Can you work these out from the model? Positions are in its coordinate system, mm. Face numbers are marked on the shaded views. A direction names the side the tool comes from. Give positions to 0.01 mm unless a question says otherwise; leave off trailing zeros. Loops run counter-clockwise (first coordinate to the right, second up) from the corner with the lowest first, then second, coordinate; pieces in that order, holes last. Notation, with made-up numbers: (28, 85) - (59, 85) arc R30 ccw to (59, 110) - close; hole circle Ø10 at (-0.5, 76). An arc over 180 degrees is marked (long way). Answer in a Markdown table with one row per item.
from build123d import *

# Parameters (mm, degrees)
SKETCH1_R                 = 1.75
BASE_DEPTH                = 2
SKETCH2_W                 = 7
SKETCH2_H                 = 16
SIDE_BATTERY_GUIDES_DEPTH = 14
CUT_EXTRUDE1_DEPTH        = 50.658836072
SKETCH5_W                 = 15
SKETCH5_H                 = 2.5
BOSS_EXTRUDE3_DEPTH       = 6
CUT_EXTRUDE2_DEPTH        = 44.33589736
FILLET2_R                 = 2
SKETCH7_R                 = 1.6
CUT_EXTRUDE3_DEPTH        = 44.33589736
SKETCH8_W                 = 26
SKETCH8_H                 = 18
SKETCH8_R                 = 1.75
PINOUT_BD_HOLDER_DEPTH    = 2
WEIGH_REDUCER_DEPTH       = 53.318734694
FILLET3_R                 = 4
FILLET4_R                 = 2
FILLET5_DEPTH             = 2
FILLET5_START             = -7.5
FILLET5_2_DEPTH           = 15
FILLET5_START_2           = -1
FILLET5_3_DEPTH           = 4


with BuildPart() as part:
    # Sketch1 → base (new body)
    with BuildSketch(Plane(origin=(0, 0, 0), x_dir=(1, 0, 0), z_dir=(0, 1, 0))):
        with BuildLine():
            Line((-25, 29), (25, 29))
            ThreePointArc((25, 29), (27.828427125, 27.828427125), (29, 25))
            Line((29, 25), (29, -25))
            ThreePointArc((29, -25), (27.828427125, -27.828427125), (25, -29))
            Line((25, -29), (-25, -29))
            ThreePointArc((-25, -29), (-27.828427125, -27.828427125), (-29, -25))
            Line((-29, -25), (-29, 25))
            ThreePointArc((-29, 25), (-27.828427125, 27.828427125), (-25, 29))
        make_face()
        with Locations(Location((23.75, 23.75, 0), (0, 0, 270))):
            Circle(SKETCH1_R, mode=Mode.SUBTRACT)
        with Locations(Location((23.75, -23.75, 0), (0, 0, 270))):
            Circle(SKETCH1_R, mode=Mode.SUBTRACT)
        with Locations(Location((-23.75, -23.75, 0), (0, 0, 270))):
            Circle(SKETCH1_R, mode=Mode.SUBTRACT)
        with Locations(Location((-23.75, 23.75, 0), (0, 0, 270))):
            Circle(SKETCH1_R, mode=Mode.SUBTRACT)
        with BuildLine():
            Line((-11, 13), (11, 13))
            ThreePointArc((11, 13), (12.414213562, 12.414213562), (13, 11))
            Line((13, 11), (13, -11))
            ThreePointArc((13, -11), (12.414213562, -12.414213562), (11, -13))
            Line((11, -13), (-11, -13))
            ThreePointArc((-11, -13), (-12.414213562, -12.414213562), (-13, -11))
            Line((-13, -11), (-13, 11))
            ThreePointArc((-13, 11), (-12.414213562, 12.414213562), (-11, 13))
        make_face(mode=Mode.SUBTRACT)
    extrude(amount=BASE_DEPTH)

    # Sketch2 → side battery guides (add)
    with BuildSketch(Plane(origin=(0, 2, 0), x_dir=(1, 0, 0), z_dir=(0, 1, 0))):
        with Locations((-22, 0)):
            Rectangle(SKETCH2_W, SKETCH2_H)
        with Locations((22, 0)):
            Rectangle(SKETCH2_W, SKETCH2_H)
    extrude(amount=SIDE_BATTERY_GUIDES_DEPTH)

    # Sketch4 → Cut-Extrude1 (cut, through all)
    with BuildSketch(Plane.XY.offset(8)):
        Polygon((-18.5, 16), (-22.5, 16), (-22.5, 8), (-18.5, 2), align=None)
        Polygon((18.5, 2), (18.5, 16), (22.5, 16), (22.5, 8), align=None)
    extrude(amount=-CUT_EXTRUDE1_DEPTH, mode=Mode.SUBTRACT)

    # Sketch5 → Boss-Extrude3 (add)
    with BuildSketch(Plane(origin=(0, 2, 0), x_dir=(1, 0, 0), z_dir=(0, 1, 0))):
        with Locations((0, 21.25)):
            Rectangle(SKETCH5_W, SKETCH5_H)
        with Locations((0, -21.25)):
            Rectangle(SKETCH5_W, SKETCH5_H)
    extrude(amount=BOSS_EXTRUDE3_DEPTH)

    # Sketch6 → Cut-Extrude2 (cut, through all)
    with BuildSketch(Plane(origin=(0, 2, 0), x_dir=(1, 0, 0), z_dir=(0, 1, 0))):
        Polygon((-25.5, 8), (-25.5, 17), (-29, 22), (-29, -22), (-25.5, -17), (-25.5, -8), align=None)
        Polygon((-15.45, -22.5), (-7.5, -22.5), (7.5, -22.5), (15.45, -22.5), (20, -29), (-20, -29), align=None)
        Polygon((29, 22), (29, -22), (25.5, -17), (25.5, -8), (25.5, 8), (25.5, 17), align=None)
        Polygon((-7.5, 22.5), (7.5, 22.5), (15.45, 22.5), (20, 29), (-20, 29), (-15.45, 22.5), align=None)
    extrude(amount=-CUT_EXTRUDE2_DEPTH, mode=Mode.SUBTRACT)

    # Fillet2
    fillet2_edges = [part.edges().sort_by_distance(p)[0] for p in [
        (-25.5, 1, -17),
        (-25.5, 1, 17),
        (-29, 1, 22),
        (-29, 1, -22),
        (-20, 1, 29),
        (-15.45, 1, 22.5),
        (15.45, 1, 22.5),
        (20, 1, 29),
        (25.5, 1, -17),
        (29, 1, -22),
        (29, 1, 22),
        (25.5, 1, 17),
        (-15.45, 1, -22.5),
        (-20, 1, -29),
        (20, 1, -29),
        (15.45, 1, -22.5),
    ]]
    fillet(fillet2_edges, radius=FILLET2_R)

    # Sketch7 → Cut-Extrude3 (cut, through all)
    with BuildSketch(Plane(origin=(0, 2, 0), x_dir=(1, 0, 0), z_dir=(0, 1, 0))):
        with Locations(Location((15.25, 15.25, 0), (0, 0, 270))):
            Circle(SKETCH7_R)
        with Locations(Location((15.25, -15.25, 0), (0, 0, 90))):
            Circle(SKETCH7_R)
        with Locations(Location((-15.25, -15.25, 0), (0, 0, 270))):
            Circle(SKETCH7_R)
        with Locations(Location((-15.25, 15.25, 0), (0, 0, 90))):
            Circle(SKETCH7_R)
    extrude(amount=-CUT_EXTRUDE3_DEPTH, mode=Mode.SUBTRACT)

    # Sketch8 → pinout_bd_holder (add)
    with BuildSketch(Plane(origin=(0, 2, 0), x_dir=(1, 0, 0), z_dir=(0, 1, 0))):
        with Locations((0, 31.5)):
            Rectangle(SKETCH8_W, SKETCH8_H)
        with Locations(Location((-10, 37, 0), (0, 0, 270))):
            Circle(SKETCH8_R, mode=Mode.SUBTRACT)
        with Locations(Location((10, 37, 0), (0, 0, 90))):
            Circle(SKETCH8_R, mode=Mode.SUBTRACT)
    extrude(amount=-PINOUT_BD_HOLDER_DEPTH)

    # Sketch9 → Weigh-Reducer (cut, through all)
    with BuildSketch(Plane.XZ):
        with BuildLine():
            Line((-7.5, -23), (7.5, -23))
            ThreePointArc((7.5, -23), (8.560660172, -23.439339828), (9, -24.5))
            Line((9, -24.5), (9, -32))
            ThreePointArc((9, -32), (8.560660172, -33.060660172), (7.5, -33.5))
            Line((7.5, -33.5), (6.5, -33.5))
            ThreePointArc((6.5, -33.5), (5.439339828, -33.939339828), (5, -35))
            Line((5, -35), (5, -36))
            ThreePointArc((5, -36), (4.560660172, -37.060660172), (3.5, -37.5))
            Line((3.5, -37.5), (-3.5, -37.5))
            ThreePointArc((-3.5, -37.5), (-4.560660172, -37.060660172), (-5, -36))
            Line((-5, -36), (-5, -35))
            ThreePointArc((-5, -35), (-5.439339828, -33.939339828), (-6.5, -33.5))
            Line((-6.5, -33.5), (-7.5, -33.5))
            ThreePointArc((-7.5, -33.5), (-8.560660172, -33.060660172), (-9, -32))
            Line((-9, -32), (-9, -24.5))
            ThreePointArc((-9, -24.5), (-8.560660172, -23.439339828), (-7.5, -23))
        make_face()
    extrude(amount=-WEIGH_REDUCER_DEPTH, mode=Mode.SUBTRACT)

    # Fillet3
    fillet3_edges = [part.edges().sort_by_distance(p)[0] for p in [
        (22.5, 8, 0),
        (-18.5, 2, 0),
        (18.5, 2, 0),
        (-22.5, 8, 0),
    ]]
    fillet(fillet3_edges, radius=FILLET3_R)

    # Fillet4
    fillet4_edges = [part.edges().sort_by_distance(p)[0] for p in [
        (0, 2, -20),
        (0, 2, 20),
    ]]
    fillet(fillet4_edges, radius=FILLET4_R)

    # Fillet5: read off the stored shape, not the designer's step
    # Fillet5 outline → Fillet5 (add)
    with BuildSketch(Plane(origin=(0, 0, 0), x_dir=(1, 0, 0), z_dir=(0, 1, 0))):
        with BuildLine():
            Line((-13, 22.5), (-13, 24.410589217))
            ThreePointArc((-13, 24.410589217), (-13.390245011, 23.223707219), (-14.408688877, 22.5))
            Line((-14.408688877, 22.5), (-13, 22.5))
        make_face()
        with BuildLine():
            ThreePointArc((14.408688877, 22.5), (13.390245011, 23.223707219), (13, 24.410589217))
            Line((13, 24.410589217), (13, 22.5))
            Line((13, 22.5), (14.408688877, 22.5))
        make_face()
    extrude(amount=FILLET5_DEPTH)

    # Fillet5 2 outline → Fillet5 2 (add)
    with BuildSketch(Plane.YZ.offset(FILLET5_START)):
        with BuildLine():
            ThreePointArc((2, -23), (2.615768875, -22.629171307), (3.322875656, -22.5))
            Line((3.322875656, -22.5), (2, -22.5))
            Line((2, -22.5), (2, -23))
        make_face()
    extrude(amount=FILLET5_2_DEPTH)

    # Fillet5 3 outline → Fillet5 3 (cut)
    with BuildSketch(Plane(origin=(0, 0, 0), x_dir=(1, 0, 0), z_dir=(0, 1, 0)).offset(FILLET5_START_2)):
        with BuildLine():
            ThreePointArc((-13, 38.5), (-12.414213562, 39.914213562), (-11, 40.5))
            Line((-11, 40.5), (-13, 40.5))
            Line((-13, 40.5), (-13, 38.5))
        make_face()
        with BuildLine():
            ThreePointArc((11, 40.5), (12.414213562, 39.914213562), (13, 38.5))
            Line((13, 38.5), (13, 40.5))
            Line((13, 40.5), (11, 40.5))
        make_face()
    extrude(amount=FILLET5_3_DEPTH, mode=Mode.SUBTRACT)


solid = part.part
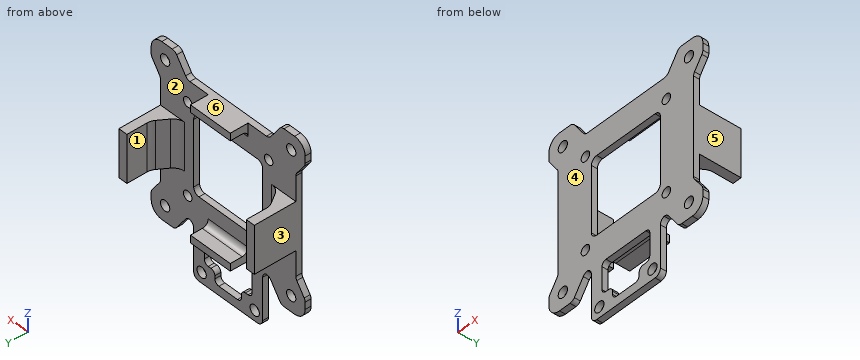
Q1. Imagine slicing it at D-D, the plane x = 10. Write out the boundary of the cut face in (y, z).
Checked values:
| item | result |
|---|---|
| outline | (0, -40.5) - (2, -40.5) - (2, -38.75) - (0, -38.75) - close; (0, -35.25) - (2, -35.25) - (2, -13) - (0, -13) - close; (0, 13) - (2, 13) - (2, 22.5) - (0, 22.5) - close |
Q2. Imagine slicing it at A-A, the plane x = -23.75. Write out the boundary of the cut face in (y, z), and give its area (3 significant figures).
Checked values:
| item | result |
|---|---|
| outline | (0, -29) - (2, -29) - (2, -25.5) - (0, -25.5) - close; (0, -22) - (2, -22) - (2, -8) - (16, -8) - (16, 8) - (2, 8) - (2, 22) - (0, 22) - close; (0, 25.5) - (2, 25.5) - (2, 29) - (0, 29) - close |
| area | 326 mm² |
Q3. If we mould it in two halves opening along X, with no side actions, what happens to the marked faces 4, 5 and 6? For each: released by +X, released by -X, zero draft, split by the parting line, or undercut.
Checked values:
| item | result |
|---|---|
| face 4 | zero draft |
| face 5 | released by +X |
| face 6 | undercut |
Q4. Imagine slicing it at C-C, the plane z = -15.25. Write out the boundary of the cut face in (x, y), and give its area (3 significant figures).
Checked values:
| item | result |
|---|---|
| outline | (-25.5, 0) - (-16.85, 0) - (-16.85, 2) - (-25.5, 2) - close; (-13.65, 0) - (13.65, 0) - (13.65, 2) - (-13.65, 2) - close; (16.85, 0) - (25.5, 0) - (25.5, 2) - (16.85, 2) - close |
| area | 89.2 mm² |
Q5. Imagine slicing it at B-B, the plane z = -6. Write out the boundary of the cut face in (x, y).
Checked values:
| item | result |
|---|---|
| outline | (-25.5, 0) - (-13, 0) - (-13, 2) - (-16.36, 2) arc R4 cw to (-19.69, 3.78) - (-21.83, 6.99) arc R4 cw to (-22.5, 9.21) - (-22.5, 16) - (-25.5, 16) - close; (13, 0) - (25.5, 0) - (25.5, 16) - (22.5, 16) - (22.5, 9.21) arc R4 cw to (21.83, 6.99) - (19.69, 3.78) arc R4 cw to (16.36, 2) - (13, 2) - close |
Q6. If I drill on line 1 (X direction, y = 0.7, z = 15.25); line 2 (X direction, y = 0.8, z = 23.75) (3 decimals); line 3 (X direction, y = 10.25, z = -3), over which ranges is the centre line in solid material (lowest first)? Write a range as [from, to].
Checked values:
| item | result |
|---|---|
| line 1 | x = [-25.5, -16.85], [-13.65, 13.65], [16.85, 25.5] |
| line 2 | x = [-29, -25.5], [-22, -16.325], [16.325, 22], [25.5, 29] |
| line 3 | x = [-25.5, -22.5], [22.5, 25.5] |
Q7. On a 3-axis mill with a long thin cutter (end or side, diameter ignored), from which of +Z, -Z, +X, -X, +Y, -Y can I reach the whole of each face in a straight line? I mean the marked faces 1, 2 and 3. Say none if no direction works.
Checked values:
| item | result |
|---|---|
| face 1 | +Z, -Z, +Y |
| face 2 | +Y |
| face 3 | -X, +Y, -Y |
Q8. For pin 1 (3.5 mm diameter, centred on y = 5.5, z = 20, fed in from -X); pin 2 (8 mm diameter, centred on x = 15.5, y = 12, fed in from -Z); pin 3 (2 mm diameter, centred on y = 3.5, z = 20, fed in from +X); pin 4 (1.2 mm diameter, centred on x = 0.5, y = 5.5, fed in from +Z), each with a flat end and sliding along its axis, tell me the tip position at first contact or that it passes through.
Checked values:
| item | result |
|---|---|
| pin 1 | stops at x = -7.5 |
| pin 2 | passes through |
| pin 3 | stops at x = 7.5 |
| pin 4 | stops at z = 22.5 |
